The model under review builds one solid part; all positions refer to its coordinate system, in mm. A direction names the side the tool comes from. Round coordinates to 2 decimals unless told otherwise and drop trailing zeros. Order: outer loops, then holes, each group sorted by start corner. A loop starts at its lowest first (then second) coordinate and runs counter-clockwise, first axis right, second up. Notation, with made-up numbers: M -38.5,51.25 L 16.5,51.25 A15 cw 16.5,70.25 Z; hole C -12,29 d3. An arc over 180 degrees is marked long. Answer as a JSON object with one key per item and string values. Group by question number.
1. Add section A-A on y = 45. State the section outline as (x, z) points, and give its area (3 significant figures).
2. Mouldability with a two-part tool opening along Y and no side actions: class faces 6 (the face through (-1, 98, 47)), 7 (the face through (78.056, 38.497, 18.713)), 8 (the face through (74, 24, 26)) as released by +Y, released by -Y, zero draft, split by the parting line, or undercut.
3. Add section C-C on z = 87. State the section outline as (x, y) points, and give its area (3 significant figures).
4. Clearance check with flat-ended pins moving along their axes: P1, Ø10, axis at x = 25, z = 42.5, coming from the -Y side; P2, Ø19.5, axis at x = -70.5, y = 62.5, coming from the -Z side. State where each tip first meets the part, or that it passes through.
5. To check wall thickness, follow probe 1 along X at (y, z) = (56.5, 91.5); probe 2 along Z at (x, y) = (76, 45); probe 3 along Y at (x, z) = (44.5, 37.5). State the ranges of each line that lie inside material, in increasing order. Write a range as [from, to].
6. Machinability: for faces 1 (the face through (75, 61, 0)), 2 (the face through (-75, 61, 0)), 3 (the face through (-1, 90, 47)), 4 (the face through (75, 61, 96)), 5 (the face through (-75, 61, 96)), which of the approach directions +Z, -Z, +X, -X, +Y, -Y give a long, thin tool a straight path to every point of the face, cutting with its end or side? Answer none if there is none.
7. Add section D-D on x = -16.5. State the section outline as (y, z) points.
8. Add section B-B on z = 48. State the section outline as (x, y) points.
```python
from build123d import *

# Parameters (mm, degrees)
EXTRUDE_1_DEPTH     = 96
SKETCH_2_R          = 30
CUT_EXTRUDE_1_DEPTH = 172
SKETCH_3_R          = 75
EXTRUDE_2_DEPTH     = 8


with BuildPart() as part:
    # 草图1 → 凸台-拉伸1 (new body)
    with BuildSketch(Plane.XY):
        Polygon((-82, 98), (82, 98), (82, 0), (74, 0), (74, 90), (-74, 90), (-74, 0), (-82, 0), align=None)
    extrude(amount=EXTRUDE_1_DEPTH)

    # 草图2 → 切除-拉伸1 (cut)
    with BuildSketch(Plane(origin=(82, 0, 0), x_dir=(0, 0, -1), z_dir=(1, 0, 0))):
        with Locations(Location((-48, 45, 0), (0, 0, 90))):
            Circle(SKETCH_2_R)
    extrude(amount=-CUT_EXTRUDE_1_DEPTH, mode=Mode.SUBTRACT)

    # 草图3 → 凸台-拉伸2 (add)
    with BuildSketch(Plane(origin=(0, 98, 0), x_dir=(1, 0, 0), z_dir=(0, 1, 0))):
        with Locations((0, -48)):
            Circle(SKETCH_3_R)
    extrude(amount=-EXTRUDE_2_DEPTH)


solid = part.part
```
Recorded:
{
 "1": {"outline": "M -82,0 L -74,0 L -74,18 L -82,18 Z; M -82,78 L -74,78 L -74,96 L -82,96 Z; M 74,0 L 82,0 L 82,18 L 74,18 Z; M 74,78 L 82,78 L 82,96 L 74,96 Z", "area": "576 mm²"},
 "2": {"face 6": "released by +Y", "face 7": "undercut", "face 8": "zero draft"},
 "3": {"outline": "M -82,0 L -74,0 L -74,90 L 74,90 L 74,0 L 82,0 L 82,98 L -82,98 Z", "area": "2,750 mm²"},
 "4": {"P1": "stops at y = 90", "P2": "stops at z = 0"},
 "5": {"probe 1": "x = [-82, -74], [74, 82]", "probe 2": "z = [0, 18], [78, 96]", "probe 3": "y = [90, 98]"},
 "6": {"face 1": "-Z, +X, +Y, -Y", "face 2": "-Z, -X, +Y, -Y", "face 3": "+Z, -Z, -Y", "face 4": "+Z, +X, +Y, -Y", "face 5": "+Z, -X, +Y, -Y"},
 "7": {"outline": "M 90,-25.16 L 98,-25.16 L 98,121.16 L 90,121.16 Z"},
 "8": {"outline": "M -82,0 L -74,0 L -74,15 L -82,15 Z; M -82,75 L -74,75 L -74,90 L 74,90 L 74,75 L 82,75 L 82,98 L -82,98 Z; M 74,0 L 82,0 L 82,15 L 74,15 Z"}
}
